The model under review builds one solid part; all positions refer to its coordinate system, in mm. A direction names the side the tool comes from. Coordinates: 2 decimals unless noted, no trailing zeros. Order: outer loops, then holes, each group sorted by start corner. A loop starts at its lowest first (then second) coordinate and runs counter-clockwise, first axis right, second up. Notation, with made-up numbers: M 46.25,88.25 L 55.25,88.25 A29 cw 55.25,111.25 Z; hole C -6.75,45.25 d3. An arc over 180 degrees is marked long. Answer in a Markdown table with one row per item.
from build123d import *

# Parameters (mm, degrees)
F1_DEPTH = 63.5
F2_DEPTH = 25.4
F3_DEPTH = 7.9375
F5_R     = 6.35


with BuildPart() as f1:
    # F0 (on Front) → F1 (new body, symmetric)
    with BuildSketch(Plane.XZ):
        Polygon((22.225, 9.525), (-41.275, 9.525), (-41.275, -9.525), (41.275, -9.525), (41.275, 9.525), align=None)
    extrude(amount=F1_DEPTH, both=True)

    # F0 (on Front) → F2 (join, symmetric)
    with BuildSketch(Plane.XZ):
        with BuildLine():
            Line((22.225, 27.0002), (22.225, 9.525))
            Line((22.225, 9.525), (41.275, 9.525))
            Line((41.275, 9.525), (41.275, 27.0002))
            ThreePointArc((41.275, 27.0002), (45.9246798487, 38.2255201513), (57.15, 42.8752))
            Line((57.15, 42.8752), (60.325, 42.8752))
            Line((60.325, 42.8752), (60.325, 61.9252))
            Line((60.325, 61.9252), (57.15, 61.9252))
            add(Edge.make_bspline(
                [(54.3975584456, 61.8165710126), (55.3245975256, 61.8674152236), (56.2423933206, 61.9037658761), (57.15, 61.9252)],
                knots=[108.931400428, 108.931400428, 108.931400428, 108.931400428, 111.5045361635, 111.5045361635, 111.5045361635, 111.5045361635], degree=3))
            ThreePointArc((54.3975584456, 61.8165710126), (31.4996135869, 50.7028011623), (22.225, 27.0002))
        make_face()
        Polygon((85.725, 61.9252), (60.325, 61.9252), (60.325, 42.8752), (85.725, 42.8752), (85.725, 52.3875), align=None)
    extrude(amount=F2_DEPTH, both=True)

    # F0 (on Front) → F3 (join, symmetric)
    with BuildSketch(Plane.XZ):
        with BuildLine():
            add(Edge.make_bspline(
                [(-41.275, 9.525), (-40.658780826, 31.5366673239), (15.1521879644, 59.6641268054), (54.3975584456, 61.8165710126)],
                knots=[0, 0, 0, 0, 108.931400428, 108.931400428, 108.931400428, 108.931400428], degree=3))
            Line((-41.275, 9.525), (22.225, 9.525))
            Line((22.225, 9.525), (22.225, 27.0002))
            ThreePointArc((22.225, 27.0002), (31.4996135869, 50.7028011623), (54.3975584456, 61.8165710126))
        make_face()
    extrude(amount=F3_DEPTH, both=True)

    # F0 (on Front) → F4 (revolve)
    with BuildSketch(Plane.XZ):
        Polygon((85.725, 66.675), (85.725, 61.9252), (85.725, 52.3875), (85.725, 42.8752), (85.725, 38.1), (111.125, 38.1), (111.125, 66.675), align=None)
    revolve(axis=Axis((85.725, 0, 45.24375), (0, 0, -1)))

    # F5
    f5_edges = [f1.edges().sort_by_distance(p)[0] for p in [
        (-41.275, -63.5, 0),
        (41.275, -63.5, 0),
        (41.275, 63.5, 0),
        (-41.275, 63.5, 0),
    ]]
    fillet(f5_edges, radius=F5_R)


solid = f1.part
(1) Insertion check: P1, Ø6, axis at x = -5.5, y = 39, coming from the +Z side (3 decimals); P2, Ø19, axis at y = -16.5, z = 16, coming from the -X side (3 decimals); P3, Ø14.5, axis at x = 65.5, y = 8.5, coming from the -Z side; P4, Ø5, axis at y = 19, z = 20.5, coming from the -X side (3 decimals). Each pin has a flat end and moves straight along its axis. Give the tip position at first contact, or say it passes through.
Report:
| item | result |
|---|---|
| P1 | z = 9.525 |
| P2 | x = -41.275 |
| P3 | z = 38.1 |
| P4 | x = 22.225 |
(2) To check wall thickness, follow line 1 (Z direction, x = -33, y = 45.5) (3 decimals); line 2 (Y direction, x = 22.5, z = 48); line 3 (Z direction, x = 70.5, y = -2) (3 decimals). State the ranges of each line that lie inside material, in increasing order. Write a range as [from, to].
Report:
| item | result |
|---|---|
| line 1 | [-9.525, 9.525] |
| line 2 | [-7.94, 7.94] |
| line 3 | [38.1, 66.675] |
(3) Take a section at A-A (y = -40). Write out the cut boundary in (x, z) (3 decimals).
Report:
| item | result |
|---|---|
| outline | M -41.275,-9.525 L 41.275,-9.525 L 41.275,9.525 L -41.275,9.525 Z |
(4) Machinability: for faces 1 (the flat face through (46, 25.4, 42)), 2 (the cylindrical face through (31.75, -16.79, 50.97)), 3 (the flat face through (-3, 7.938, 30)), 4 (the flat face through (41.275, -1, 4)), which of the approach directions +Z, -Z, +X, -X, +Y, -Y give a long, thin tool a straight path to every point of the face, cutting with its end or side? Answer none if there is none.
Report:
| item | result |
|---|---|
| face 1 | +Z, +X, -X, +Y |
| face 2 | +Z, -X, -Y |
| face 3 | +Z, -X, +Y |
| face 4 | -Z, +X, +Y, -Y |
